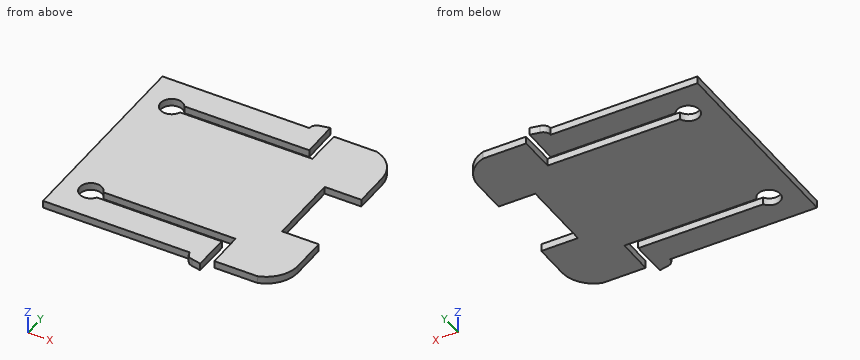
```python
from build123d import *

# Parameters (mm, degrees)
F1_DEPTH = 1


with BuildPart() as f1:
    # F0 (on Top) → F1 (new body)
    with BuildSketch(Plane.XY):
        with BuildLine():
            Line((12.941082, 13.656496), (7.447495, 13.656496))
            Line((7.447495, 13.656496), (7.417744, 8.656584))
            Line((7.417744, 8.656584), (-10.582252, 8.64454))
            ThreePointArc((-10.582252, 8.64454), (-13.493531, 8.959871), (-10.723445, 9.909398))
            Line((-10.723445, 9.909398), (6.276555, 9.910218))
            Line((6.276555, 9.910218), (6.230077, 14.910002))
            Line((6.230077, 14.910002), (5.003915, 14.656496))
            ThreePointArc((5.003915, 14.656496), (4.365699, 14.327975), (4.112004, 13.656496))
            Line((4.112004, 13.656496), (-15.887996, 13.656496))
            Line((-15.887996, 13.656496), (-15.887996, -14.343504))
            Line((-15.887996, -14.343504), (4.112004, -14.343504))
            ThreePointArc((4.112004, -14.343504), (4.365699, -15.014984), (5.003915, -15.343504))
            Line((5.003915, -15.343504), (6.230077, -15.597011))
            Line((6.230077, -15.597011), (6.276555, -10.597227))
            Line((6.276555, -10.597227), (-10.723445, -10.596407))
            ThreePointArc((-10.723445, -10.596407), (-13.493531, -9.646879), (-10.582252, -9.331549))
            Line((-10.582252, -9.331549), (7.417744, -9.343593))
            Line((7.417744, -9.343593), (7.447495, -14.343504))
            Line((7.447495, -14.343504), (13.294204, -14.343504))
            ThreePointArc((13.294204, -14.343504), (15.554923, -12.77892), (16.424473, -10.17073))
            Line((16.424473, -10.17073), (16.424473, -5.343504))
            Line((16.424473, -5.343504), (11.424473, -5.343504))
            Line((11.424473, -5.343504), (11.424473, 4.656496))
            Line((11.424473, 4.656496), (12.941082, 4.656496))
            Line((12.941082, 4.656496), (12.941082, 13.656496))
        make_face()
        with BuildLine():
            Line((13.294204, 13.656496), (12.941082, 13.656496))
            Line((12.941082, 13.656496), (12.941082, 4.656496))
            Line((12.941082, 4.656496), (16.424473, 4.656496))
            Line((16.424473, 4.656496), (16.424473, 9.483721))
            ThreePointArc((16.424473, 9.483721), (15.554923, 12.091912), (13.294204, 13.656496))
        make_face()
    extrude(amount=F1_DEPTH)


solid = f1.part
```
Verification items for the finished model (mm, model axes). Round coordinates to 2 decimals unless told otherwise and drop trailing zeros. Order: outer loops, then holes, each group sorted by start corner. A loop starts at its lowest first (then second) coordinate and runs counter-clockwise, first axis right, second up. Notation, with made-up numbers: (25, 87) - (53, 87) arc R13 cw to (53, 95) - close; hole circle Ø4 at (27.5, 71.25). An arc over 180 degrees is marked (long way). Use CSV: the item, a comma, the result in double quotes. Start each with the question number.
1) Thickness scan on L1, parallel to Y at x = -3, z = 0.45; L2, parallel to X at y = -3.5, z = 0.95. Record the ranges inside material, lowest first.
2) Section check B-B, the plane z = 0.4. Record the cut outline in (x, y), plus the area to 3 significant figures.
3) Section check A-A, the plane x = -13. Record the cut outline in (y, z), plus the area to 3 significant figures.
4) Section check D-D, the plane y = 2.5. Record the cut outline in (x, z), plus the area to 3 significant figures.
5) Section check C-C, the plane x = -8. Record the cut outline in (y, z), plus the area to 3 significant figures.
6) Go/stop test with flat-tipped pins: P1, Ø0.5, axis at x = -2, z = 0.5, coming from the +Y side; P2, Ø1.8, axis at x = -12, y = 9.13, coming from the +Z side; P3, Ø0.5, axis at x = 14.5, z = 0.5, coming from the -Y side. Record where each tip stops, or that it passes through.
Answers:
1,L1,"y = -14.34 to -10.6, -9.34 to 8.65, 9.91 to 13.66"
1,L2,"x = -15.89 to 11.42"
2,outline,"(-15.89, -14.34) - (4.11, -14.34) arc R1 ccw to (5, -15.34) - (6.23, -15.6) - (6.28, -10.6) - (-10.72, -10.6) arc R1.5 cw (long way) to (-10.58, -9.33) - (7.42, -9.34) - (7.45, -14.34) - (13.29, -14.34) arc R4.35 ccw to (16.42, -10.17) - (16.42, -5.34) - (11.42, -5.34) - (11.42, 4.66) - (16.42, 4.66) - (16.42, 9.48) arc R4.35 ccw to (13.29, 13.66) - (7.45, 13.66) - (7.42, 8.66) - (-10.58, 8.64) arc R1.5 cw (long way) to (-10.72, 9.91) - (6.28, 9.91) - (6.23, 14.91) - (5, 14.66) arc R1 ccw to (4.11, 13.66) - (-15.89, 13.66) - close"
2,area,"784 mm²"
3,outline,"(-14.34, 0) - (-10.93, 0) - (-10.93, 1) - (-14.34, 1) - close; (-8.69, 0) - (8.01, 0) - (8.01, 1) - (-8.69, 1) - close; (10.25, 0) - (13.66, 0) - (13.66, 1) - (10.25, 1) - close"
3,area,"23.5 mm²"
4,outline,"(-15.89, 0) - (11.42, 0) - (11.42, 1) - (-15.89, 1) - close"
4,area,"27.3 mm²"
5,outline,"(-14.34, 0) - (-10.6, 0) - (-10.6, 1) - (-14.34, 1) - close; (-9.33, 0) - (8.65, 0) - (8.65, 1) - (-9.33, 1) - close; (9.91, 0) - (13.66, 0) - (13.66, 1) - (9.91, 1) - close"
5,area,"25.5 mm²"
6,P1,"stops at y = 13.66"
6,P2,"passes through"
6,P3,"stops at y = -13.94"
